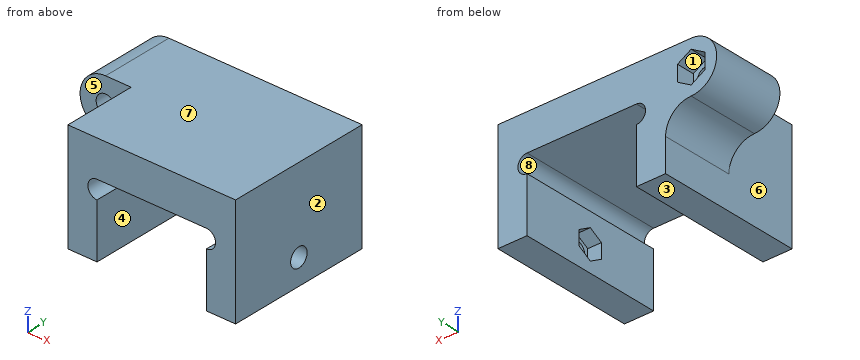
```python
from build123d import *

# Parameters (mm, degrees)
F0_R     = 3.302
F1_DEPTH = 50.8
F3_DEPTH = 38.101
F4_R     = 3.302
F5_DEPTH = 6.35
F6_R     = 3.302
F7_DEPTH = 10.16
F9_DEPTH = 4.7625


with BuildPart() as f1:
    # F0 (on Front) → F1 (new body)
    with BuildSketch(Plane.XZ):
        with BuildLine():
            Line((0, 11.43), (0, 0))
            Line((0, 0), (10.16, 0))
            Line((10.16, 0), (10.16, 19.05))
            ThreePointArc((10.16, 19.05), (6.985, 22.225), (10.16, 25.4))
            Line((10.16, 25.4), (48.26, 25.4))
            ThreePointArc((48.26, 25.4), (51.435, 22.225), (48.26, 19.05))
            Line((48.26, 19.05), (48.26, 0))
            Line((48.26, 0), (58.42, 0))
            Line((58.42, 0), (58.42, 38.1))
            Line((58.42, 38.1), (-8.89, 38.1))
            ThreePointArc((-8.89, 38.1), (-17.78, 29.21), (-8.89, 20.32))
            ThreePointArc((-8.89, 20.32), (-2.603821, 17.716179), (0, 11.43))
        make_face()
        with Locations((-8.89, 29.21)):
            Circle(F0_R, mode=Mode.SUBTRACT)
    extrude(amount=F1_DEPTH)

    # F2 (on face) → F3 (cut, through all)
    with BuildSketch(Plane(origin=(0, 0, 0), x_dir=(1, 0, 0), z_dir=(0, 0, -1))):
        Polygon((0, 50.8), (-8.89, 50.8), (-17.78, 50.8), (-17.78, 25.4), (0, 25.4), align=None)
    extrude(amount=-F3_DEPTH, mode=Mode.SUBTRACT)

    # F4 (on face) → F5 (cut)
    with BuildSketch(Plane(origin=(0, 0, 0), x_dir=(-1, 0, 0), z_dir=(0, 1, 0))):
        Polygon((13.6525, 26.460369), (13.6525, 31.959631), (8.89, 34.709261), (4.1275, 31.959631), (4.1275, 26.460369), (8.89, 23.710739), align=None)
        with Locations((8.89, 29.21)):
            Circle(F4_R, mode=Mode.SUBTRACT)
    extrude(amount=-F5_DEPTH, mode=Mode.SUBTRACT)

    # F6 (on face) → F7 (cut, through all)
    with BuildSketch(Plane.YZ.offset(58.42)):
        with Locations((-25.4, 8.89)):
            Circle(F6_R)
    extrude(amount=-F7_DEPTH, mode=Mode.SUBTRACT)

    # F8 (on face) → F9 (cut)
    with BuildSketch(Plane(origin=(48.26, 0, 0), x_dir=(0, -1, 0), z_dir=(-1, 0, 0))):
        Polygon((29.845, 11.456322), (25.4, 14.022644), (20.955, 11.456322), (20.955, 6.323678), (25.4, 3.757356), (29.845, 6.323678), align=None)
    extrude(amount=-F9_DEPTH, mode=Mode.SUBTRACT)


solid = f1.part
```
Can you work these out from the model? Positions are in its coordinate system, mm. Face numbers are marked on the shaded views. A direction names the side the tool comes from. Coordinates: 2 decimals unless noted, no trailing zeros. Loops run counter-clockwise (first coordinate to the right, second up) from the corner with the lowest first, then second, coordinate; pieces in that order, holes last.
1) Which directions (+Z, -Z, +X, -X, +Y, -Y) give clear straight access to the entire face, cutting with the end or side of a thin tool? Please do the marked faces 4, 5, 6, 7 and 8.
2) Thinking about a two-plate mould opening in X: for the marked faces 1, 2 and 3, which applies, pulls with the +X half, pulls with the -X half, needs draft (parallel to the pull), parting line crosses it, or undercut?
3) Imagine slicing it at D-D on x = -11. List the corners of the cut face in (y, z) for me.
4) Imagine slicing it at B-B on z = 8.89. List the corners of the cut face in (x, y) for me (1 decimal), plus the area to 3 significant figures.
5) Imagine slicing it at A-A on z = 29.21. List the corners of the cut face in (x, y) for me, plus the area to 3 significant figures.
6) I need wall thicknesses on probe 1 along X at (y, z) = (-10.5, 29.21); probe 2 along X at (y, z) = (-41.5, 16.5); probe 3 along Z at (x, y) = (48.5, -3). Which ranges of each line are inside material? Lowest first, please.
7) Imagine slicing it at C-C on y = -16.5. List the corners of the cut face in (x, z) for me (3 decimals).
8) For pin 1 (9.5 mm diameter, centred on y = -14.5, z = 6, fed in from -X); pin 2 (19 mm diameter, centred on x = 38.5, y = -26, fed in from -Z); pin 3 (5.5 mm diameter, centred on x = -12, z = 21.5, fed in from -Y), each with a flat end and sliding along its axis, tell me the tip position at first contact or that it passes through.
Completed:
1. face 4: -Z, +Y, -Y
1. face 5: +Z, -Z, -X, -Y
1. face 6: -Z, -X, -Y
1. face 7: +Z, +X, -X, +Y, -Y
1. face 8: +Y, -Y
2. face 1: undercut
2. face 2: pulls with the +X half
2. face 3: needs draft
3. outline: (-25.4, 20.57) - (0, 20.57) - (0, 24.93) - (-6.35, 24.93) - (-6.35, 26.67) - (-25.4, 26.67) - close; (-25.4, 31.75) - (-6.35, 31.75) - (-6.35, 33.49) - (0, 33.49) - (0, 37.85) - (-25.4, 37.85) - close
4. outline: (0, -50.8) - (10.2, -50.8) - (10.2, 0) - (0, 0) - close; (48.3, -50.8) - (58.4, -50.8) - (58.4, -28.7) - (53, -28.7) - (53, -29.8) - (48.3, -29.8) - close; (48.3, -21) - (53, -21) - (53, -22.1) - (58.4, -22.1) - (58.4, 0) - (48.3, 0) - close
4. area: 954 mm2
5. outline: (-17.78, -25.4) - (-12.19, -25.4) - (-12.19, -6.35) - (-13.65, -6.35) - (-13.65, 0) - (-17.78, 0) - close; (-5.59, -25.4) - (0, -25.4) - (0, -50.8) - (58.42, -50.8) - (58.42, 0) - (-4.13, 0) - (-4.13, -6.35) - (-5.59, -6.35) - close
5. area: 3,230 mm2
6. probe 1: x = -17.78 to -12.19, -5.59 to 58.42
6. probe 2: x = 0 to 10.16, 48.26 to 58.42
6. probe 3: z = 0 to 19.06, 25.39 to 38.1
7. outline: (-8.89, 20.32) arc R8.89 cw to (0, 11.43) - (0, 0) - (10.16, 0) - (10.16, 19.05) arc R3.175 cw to (10.16, 25.4) - (48.26, 25.4) arc R3.175 cw to (48.26, 19.05) - (48.26, 0) - (58.42, 0) - (58.42, 38.1) - (-8.89, 38.1) arc R8.89 ccw to start; hole circle Ø6.604 at (-8.89, 29.21)
8. pin 1: stops at x = 0
8. pin 2: stops at z = 25.4
8. pin 3: stops at y = -25.4
